The model under review builds one solid part; all positions refer to its coordinate system, in mm. A direction names the side the tool comes from. Coordinates: 2 decimals unless noted, no trailing zeros. Write each loop counter-clockwise with the first axis right and the second up, starting at its lowest first coordinate (ties: lowest second). Pieces come first, ordered by that corner, then holes. Notation, with made-up numbers: (-32, 32.25) - (9, 32.25) arc R12 cw to (9, 45.25) - close; hole circle Ø11 at (38, 44.5). An arc over 180 degrees is marked (long way). Put each result on its own line as item: value.
from build123d import *

# Parameters (mm, degrees)
SKETCH1_W           = 82
SKETCH1_H           = 82
BOSS_EXTRUDE1_DEPTH = 5
SKETCH2_W           = 78.2
SKETCH2_H           = 78.2
BOSS_EXTRUDE2_DEPTH = 5.5
SKETCH3_R           = 3
CUT_EXTRUDE1_DEPTH  = 8


with BuildPart() as part:
    # Sketch1 → Boss-Extrude1 (new body)
    with BuildSketch(Plane(origin=(0, 0, 0), x_dir=(1, 0, 0), z_dir=(0, 1, 0))):
        Rectangle(SKETCH1_W, SKETCH1_H)
    extrude(amount=BOSS_EXTRUDE1_DEPTH)

    # Sketch2 → Boss-Extrude2 (add)
    with BuildSketch(Plane(origin=(0, 5, 0), x_dir=(1, 0, 0), z_dir=(0, 1, 0))):
        Rectangle(SKETCH2_W, SKETCH2_H)
    extrude(amount=BOSS_EXTRUDE2_DEPTH)

    # Sketch3 → Cut-Extrude1 (cut)
    with BuildSketch(Plane(origin=(0, 10.5, 0), x_dir=(1, 0, 0), z_dir=(0, 1, 0))):
        with Locations(Location((-25, 25, 0), (0, 0, 270))):
            Circle(SKETCH3_R)
        with Locations(Location((-25, -25, 0), (0, 0, 90))):
            Circle(SKETCH3_R)
        with Locations(Location((25, -25, 0), (0, 0, 270))):
            Circle(SKETCH3_R)
        with Locations(Location((25, 25, 0), (0, 0, 90))):
            Circle(SKETCH3_R)
    extrude(amount=-CUT_EXTRUDE1_DEPTH, mode=Mode.SUBTRACT)


solid = part.part
1. Consider section B-B on x = -6.5. State the section outline as (y, z) points.
Determined:
outline: (0, -41) - (5, -41) - (5, -39.1) - (10.5, -39.1) - (10.5, 39.1) - (5, 39.1) - (5, 41) - (0, 41) - close
2. For pin 1 Ø5.5 at (x, z) = (25, -25) entering from +Y; pin 2 Ø3 at (x, y) = (0, 7.5) entering from -Z; pin 3 Ø4.5 at (y, z) = (8, -1) entering from +X, all flat-tipped, find the tip position at first contact; note any pin that passes through.
Determined:
pin 1: stops at y = 2.5
pin 2: stops at z = -39.1
pin 3: stops at x = 39.1
3. To check wall thickness, follow probe 1 along X at (y, z) = (8.5, 25); probe 2 along Z at (x, y) = (-23, 4.75); probe 3 along X at (y, z) = (8, 37.5). State the ranges of each line that lie inside material, in increasing order.
Determined:
probe 1: x = -39.1 to -28, -22 to 22, 28 to 39.1
probe 2: z = -41 to -27.24, -22.76 to 22.76, 27.24 to 41
probe 3: x = -39.1 to 39.1
4. The part is to be moulded in two halves that separate along X. For faces 1 (the flat face through (41, 2, 1)), 2 (the flat face through (-39.1, 8, 1)), 3 (the flat face through (25, 2.5, -25)), 4 (the flat face through (-1, 2, -41)), say which applies: +X half, -X half, draft (parallel to the pull), parting line (faces both ways), or undercut.
Determined:
face 1: +X half
face 2: -X half
face 3: undercut
face 4: draft
5. Machinability: for faces 5 (the flat face through (-25, 2.5, -25)), 6 (the flat face through (-1, 8, -39.1)), 7 (the flat face through (39.1, 8, 1)), 8 (the flat face through (-1, 8, 39.1)), which of the approach directions +Z, -Z, +X, -X, +Y, -Y give a long, thin tool a straight path to every point of the face, cutting with its end or side? Answer none if there is none.
Determined:
face 5: +Y
face 6: -Z, +X, -X, +Y
face 7: +Z, -Z, +X, +Y
face 8: +Z, +X, -X, +Y
6. Consider section A-A on y = 8. State the section outline as (x, z) points, plus the area to 3 significant figures.
Determined:
outline: (-39.1, -39.1) - (39.1, -39.1) - (39.1, 39.1) - (-39.1, 39.1) - close; hole circle Ø6 at (-25, -25); hole circle Ø6 at (-25, 25); hole circle Ø6 at (25, -25); hole circle Ø6 at (25, 25)
area: 6,000 mm^2
7. Consider section C-C on z = -25. State the section outline as (x, y) points.
Determined:
outline: (-41, 0) - (41, 0) - (41, 5) - (39.1, 5) - (39.1, 10.5) - (28, 10.5) - (28, 2.5) - (22, 2.5) - (22, 10.5) - (-22, 10.5) - (-22, 2.5) - (-28, 2.5) - (-28, 10.5) - (-39.1, 10.5) - (-39.1, 5) - (-41, 5) - close
8. Consider section D-D on x = -25. State the section outline as (y, z) points, plus the area to 3 significant figures.
Determined:
outline: (0, -41) - (5, -41) - (5, -39.1) - (10.5, -39.1) - (10.5, -28) - (2.5, -28) - (2.5, -22) - (10.5, -22) - (10.5, 22) - (2.5, 22) - (2.5, 28) - (10.5, 28) - (10.5, 39.1) - (5, 39.1) - (5, 41) - (0, 41) - close
area: 744 mm^2
